Geometry check sheet. Reference: drawing and pictorial views, mm from the part's lowest x, y, z. A direction names the side the tool comes from. Give positions to 0.01 mm unless a question says otherwise; leave off trailing zeros. Order: outer loops, then holes, each group sorted by start corner. A loop starts at its lowest first (then second) coordinate and runs counter-clockwise, first axis right, second up.
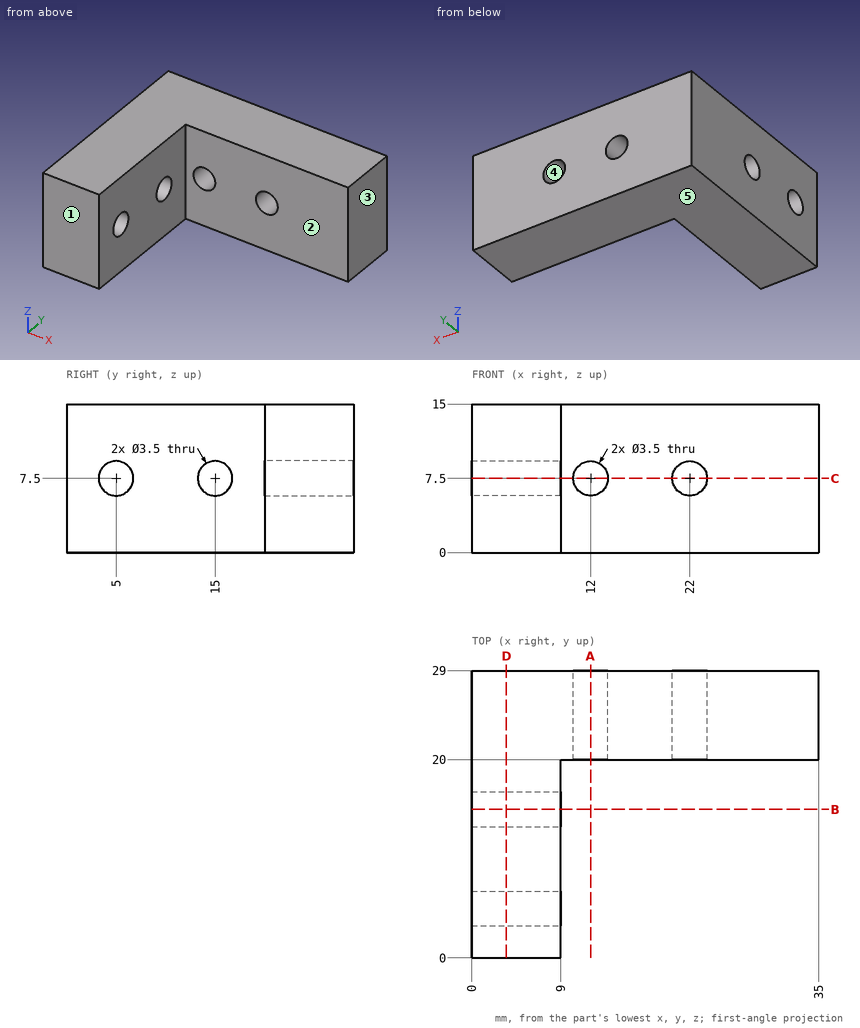
1) Material ranges on L1, parallel to Y at x = 5.75, z = 7.5; L2, parallel to X at y = 25, z = 7.5; L3, parallel to Y at x = 4, z = 8.5, recorded low to high.
Recorded:
L1: y = 0 to 3.25, 6.75 to 13.25, 16.75 to 29
L2: x = 0 to 10.25, 13.75 to 20.25, 23.75 to 35
L3: y = 0 to 3.56, 6.44 to 13.56, 16.44 to 29
2) Section check D-D, the plane x = 3.5. Record the cut outline in (y, z).
Recorded:
outline: (0, 0) - (29, 0) - (29, 15) - (0, 15) - close; hole circle Ø3.5 at (5, 7.5); hole circle Ø3.5 at (15, 7.5)
3) Section check C-C, the plane z = 7.5. Record the cut outline in (x, y).
Recorded:
outline: (0, 0) - (9, 0) - (9, 3.25) - (0, 3.25) - close; (0, 6.75) - (9, 6.75) - (9, 13.25) - (0, 13.25) - close; (0, 16.75) - (9, 16.75) - (9, 20) - (10.25, 20) - (10.25, 29) - (0, 29) - close; (13.75, 20) - (20.25, 20) - (20.25, 29) - (13.75, 29) - close; (23.75, 20) - (35, 20) - (35, 29) - (23.75, 29) - close
4) Depth check by flat-ended pin: pin 1 Ø5.5 at (x, z) = (22, 7.5) entering from -Y; pin 2 Ø8 at (x, z) = (4.5, 2.5) entering from -Y; pin 3 Ø8 at (y, z) = (9.5, 2) entering from +X; pin 4 Ø3 at (y, z) = (5, 7.5) entering from +X. Enter the tip coordinate at first touch or a pass-through.
Recorded:
pin 1: stops at y = 20
pin 2: stops at y = 0
pin 3: stops at x = 9
pin 4: passes through
5) Section check A-A, the plane x = 12. Record the cut outline in (y, z).
Recorded:
outline: (20, 0) - (29, 0) - (29, 5.75) - (20, 5.75) - close; (20, 9.25) - (29, 9.25) - (29, 15) - (20, 15) - close
6) Set-up check for the marked faces 1 and 2: record each of +Z, -Z, +X, -X, +Y, -Y from which the full face is reachable in a straight line by a thin tool's end or side.
Recorded:
face 1: +Z, -Z, +X, -X, -Y
face 2: +Z, -Z, +X, -Y
7) Section check B-B, the plane y = 15. Record the cut outline in (x, z), then the cut area to 4 significant figures.
Recorded:
outline: (0, 0) - (9, 0) - (9, 5.75) - (0, 5.75) - close; (0, 9.25) - (9, 9.25) - (9, 15) - (0, 15) - close
area: 103.5 mm2
8) Draft check along X on the marked faces 3, 4 and 5. Enter one of: +X half, -X half, draft (parallel to the pull), parting line (faces both ways), or undercut.
Recorded:
face 3: +X half
face 4: undercut
face 5: draft
